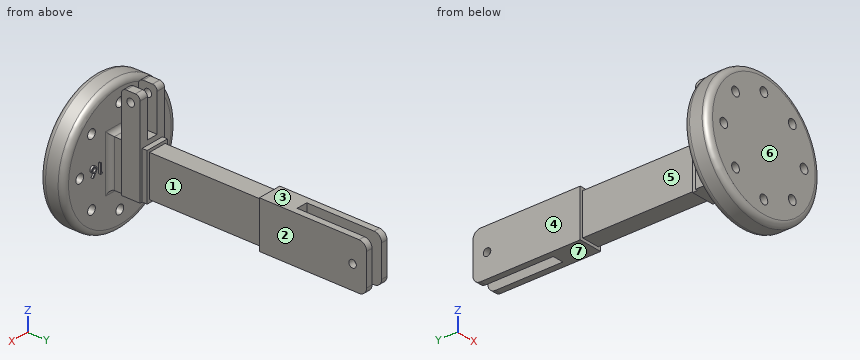
```python
from build123d import *

# Parameters (mm, degrees)
SKETCH1_W               = 70
SKETCH1_H               = 70
BOSS_EXTRUDE1_DEPTH     = 12.7
SKETCH2_R               = 2
BOSS_EXTRUDE2_DEPTH     = 6.35
CUT_EXTRUDE2_DEPTH      = 158.955689989
CUT_EXTRUDE2_DEPTH_BACK = 12.7
SKETCH3_R               = 2.413
SKETCH4_R               = 2.032
BOSS_EXTRUDE4_DEPTH     = 7.6
CUT_EXTRUDE3_DEPTH      = 12.45
SKETCH6_W               = 6
SKETCH6_H               = 36
SKETCH6_H_2             = 4
CUT_EXTRUDE4_DEPTH      = 162.187003198
BOSS_EXTRUDE5_DEPTH     = 1
SKETCH8_OUTSIDE_W       = 108.142
SKETCH8_OUTSIDE_H       = 110.642
SKETCH8_OUTSIDE_R       = 35
CUT_EXTRUDE5_DEPTH      = 147.569232812
FILLET2_R               = 3
CUT_EXTRUDE6_START      = 20
SKETCH9_OUTSIDE_W       = 108.142
SKETCH9_OUTSIDE_H       = 110.642
SKETCH9_OUTSIDE_W_2     = 9.7
SKETCH9_OUTSIDE_H_2     = 22
CUT_EXTRUDE6_DEPTH      = 60
FILLET1_R               = 2.5


with BuildPart() as part:
    # Sketch1 → Boss-Extrude1 (new body)
    with BuildSketch(Plane(origin=(0, 0, 0), x_dir=(1, 0, 0), z_dir=(0, 1, 0))):
        Rectangle(SKETCH1_W, SKETCH1_H)
    extrude(amount=BOSS_EXTRUDE1_DEPTH)

    # Sketch2 → Boss-Extrude2 (add, symmetric)
    with BuildSketch(Plane(origin=(0, 0, 0), x_dir=(0, 0, -1), z_dir=(1, 0, 0))):
        with BuildLine():
            Line((-12.5, 0), (12.5, 0))
            Line((12.5, 0), (12.5, 146))
            ThreePointArc((12.5, 146), (11.328427125, 148.828427125), (8.5, 150))
            Line((8.5, 150), (-8.5, 150))
            ThreePointArc((-8.5, 150), (-11.328427125, 148.828427125), (-12.5, 146))
            Line((-12.5, 146), (-12.5, 0))
        make_face()
        with Locations((0, 142.5)):
            Circle(SKETCH2_R, mode=Mode.SUBTRACT)
    extrude(amount=BOSS_EXTRUDE2_DEPTH, both=True)

    # Sketch3 → Cut-Extrude2 (cut, two sides: drawn at the far end of the back side and taken through both)
    with BuildSketch(Plane(origin=(0, 0, 0), x_dir=(1, 0, 0), z_dir=(0, 1, 0)).offset(-CUT_EXTRUDE2_DEPTH_BACK)):
        with Locations(Location((17.67766953, -17.67766953, 0), (0, 0, 270))):
            Circle(SKETCH3_R)
        with Locations(Location((25, 0, 0), (0, 0, 270))):
            Circle(SKETCH3_R)
        with Locations(Location((17.67766953, 17.67766953, 0), (0, 0, 270))):
            Circle(SKETCH3_R)
        with Locations(Location((0, 25, 0), (0, 0, 270))):
            Circle(SKETCH3_R)
        with Locations(Location((-17.67766953, 17.67766953, 0), (0, 0, 270))):
            Circle(SKETCH3_R)
        with Locations(Location((-25, 0, 0), (0, 0, 270))):
            Circle(SKETCH3_R)
        with Locations(Location((-17.67766953, -17.67766953, 0), (0, 0, 270))):
            Circle(SKETCH3_R)
        with Locations(Location((0, -25, 0), (0, 0, 270))):
            Circle(SKETCH3_R)
    extrude(amount=CUT_EXTRUDE2_DEPTH + CUT_EXTRUDE2_DEPTH_BACK, mode=Mode.SUBTRACT)

    # Sketch4 → Boss-Extrude4 (add, symmetric)
    with BuildSketch(Plane(origin=(0, 0, 0), x_dir=(0, 0, -1), z_dir=(1, 0, 0))):
        with BuildLine():
            Line((12.5, 20), (-35, 20))
            ThreePointArc((-35, 20), (-36.767766953, 20.732233047), (-37.5, 22.5))
            Line((-37.5, 22.5), (-37.5, 27.5))
            ThreePointArc((-37.5, 27.5), (-36.767766953, 29.267766953), (-35, 30))
            Line((-35, 30), (12.5, 30))
            Line((12.5, 30), (12.5, 20))
        make_face()
        with Locations(Location((-32.5, 25, 0), (0, 0, 180))):
            Circle(SKETCH4_R, mode=Mode.SUBTRACT)
    extrude(amount=BOSS_EXTRUDE4_DEPTH, both=True)

    # Sketch5 → Cut-Extrude3 (cut)
    with BuildSketch(Plane(origin=(0, 30, 0), x_dir=(1, 0, 0), z_dir=(0, 1, 0))):
        Polygon((-3.070505438, -14.989300838), (-3.070505438, -44.384490964), (3.070505438, -44.384490964), (2.929494562, -14.989300838), align=None)
    extrude(amount=-CUT_EXTRUDE3_DEPTH, mode=Mode.SUBTRACT)

    # Sketch6 → Cut-Extrude4 (cut, through all)
    with BuildSketch(Plane.XY.offset(12.5)):
        with Locations((0, 128)):
            Rectangle(SKETCH6_W, SKETCH6_H)
        with Locations((0, 148)):
            Rectangle(SKETCH6_W, SKETCH6_H_2)
    extrude(amount=-CUT_EXTRUDE4_DEPTH, mode=Mode.SUBTRACT)

    # Sketch7 → Boss-Extrude5 (add)
    # profile 1 of 2: a face of its own
    with BuildSketch(Plane(origin=(0, 12.7, 0), x_dir=(1, 0, 0), z_dir=(0, 1, 0))):
        Polygon((12.240261351, 2.686742079), (13.218668469, 2.686742079), (13.218668469, -2.604924587), (12.743775307, -2.604924587), (12.743775307, 2.144007037), (11.929672742, 2.144007037), align=None)
    # profile 2 of 2: a face of its own
    with BuildSketch(Plane(origin=(0, 12.7, 0), x_dir=(1, 0, 0), z_dir=(0, 1, 0))):
        with BuildLine():
            Line((17.628390691, 2.82242584), (17.994100827, 2.535157878))
            Line((17.994100827, 2.535157878), (16.595922075, 0.397078618))
            add(Edge.make_bspline(
                [(16.595922075, 0.397078618), (16.68901047, 0.411916241), (16.870589909, 0.440858701), (17.05438597, 0.445633214), (17.143957264, 0.447960028)],
                knots=[0, 0, 0, 0, 1.025318673, 2, 2, 2, 2], degree=3))
            add(Edge.make_bspline(
                [(17.143957264, 0.447960028), (17.197739491, 0.446514478), (17.303608204, 0.443668956), (17.459042297, 0.421770754), (17.60840176, 0.387261358), (17.751067531, 0.336956876), (17.887551682, 0.272697364), (18.018637448, 0.195682644), (18.141860725, 0.10193596), (18.258808341, -0.002786056), (18.364985024, -0.118774831), (18.458989298, -0.241845899), (18.537951234, -0.371871041), (18.602016567, -0.508784397), (18.65176561, -0.652374921), (18.688032645, -0.802458894), (18.709470839, -0.959139809), (18.712381997, -1.065696098), (18.713860777, -1.119823425)],
                knots=[0, 0, 0, 0, 1.04369286, 2.054478336, 3.041073146, 4.015093852, 4.984733326, 5.965804835, 6.960378782, 7.985147595, 9.009457201, 10.008161701, 10.986880575, 11.956520048, 12.937015923, 13.931873656, 14.949455224, 16, 16, 16, 16], degree=3))
            add(Edge.make_bspline(
                [(18.713860777, -1.119823425), (18.711709178, -1.193876073), (18.70747534, -1.339594158), (18.665287458, -1.551830369), (18.599731804, -1.754021196), (18.506027684, -1.942938491), (18.389637653, -2.118323329), (18.247703673, -2.273725163), (18.085259352, -2.412321529), (17.901582883, -2.528219037), (17.703911973, -2.622868888), (17.496248834, -2.690852051), (17.280610172, -2.73270682), (17.134250824, -2.737954041), (17.060214943, -2.740608348)],
                knots=[0, 0, 0, 0, 1.031375318, 2.029502543, 3.004789286, 3.987476834, 4.960371455, 5.9300674, 6.912260825, 7.929083631, 8.949397511, 9.960523116, 10.96833055, 12, 12, 12, 12], degree=3))
            add(Edge.make_bspline(
                [(17.060214943, -2.740608348), (16.989009217, -2.738297846), (16.847963141, -2.733721147), (16.640480226, -2.692951218), (16.441115902, -2.626870241), (16.251266957, -2.535831986), (16.075401269, -2.420839711), (15.918063938, -2.282406265), (15.780039469, -2.123490764), (15.665173078, -1.944117858), (15.574067614, -1.751365184), (15.505744751, -1.550376865), (15.465836145, -1.341885226), (15.460259398, -1.200550646), (15.45745052, -1.12936369)],
                knots=[0, 0, 0, 0, 1.012016664, 2.004627821, 2.994792927, 3.992885782, 4.990978636, 5.973936114, 6.964471063, 7.975201453, 8.993600317, 9.990122807, 10.98767138, 12, 12, 12, 12], degree=3))
            add(Edge.make_bspline(
                [(15.45745052, -1.12936369), (15.459236753, -1.074867713), (15.462883898, -0.96359734), (15.4883495, -0.795074346), (15.529268892, -0.622639972), (15.575095098, -0.476356846), (15.62351477, -0.356520973), (15.663810872, -0.259904982), (15.713966794, -0.160480502), (15.767447978, -0.054838219), (15.829068482, 0.05429928), (15.896069523, 0.168756019), (15.970303519, 0.286711695), (16.022343527, 0.366758276), (16.048946914, 0.407678912)],
                knots=[0, 0, 0, 0, 1.173818275, 2.396712641, 3.66331629, 4.989737886, 5.693666774, 6.447286557, 7.243889047, 8.091586357, 8.998013824, 9.943181721, 10.948533338, 12, 12, 12, 12], degree=3))
            Line((16.048946914, 0.407678912), (17.628390691, 2.82242584))
        make_face()
        with BuildLine():
            add(Edge.make_bspline(
                [(17.044314503, -0.094775015), (17.004003728, -0.095951343), (16.925265074, -0.098249053), (16.80974434, -0.111591993), (16.700413591, -0.136718438), (16.595824353, -0.168719916), (16.497931993, -0.21272097), (16.406025056, -0.266169523), (16.319748133, -0.329096781), (16.240004906, -0.400611254), (16.167706129, -0.478909827), (16.105444181, -0.562774462), (16.051737695, -0.650184031), (16.008071136, -0.741868872), (15.974068283, -0.837793937), (15.949472237, -0.93751804), (15.935783828, -1.041709908), (15.933506549, -1.112365001), (15.932343683, -1.148444219)],
                knots=[0, 0, 0, 0, 1.129588631, 2.206414736, 3.251139165, 4.268635594, 5.265702196, 6.250456724, 7.242448911, 8.251968645, 9.246821453, 10.222880186, 11.173611482, 12.116736599, 13.062300278, 14.020270554, 14.989073742, 16, 16, 16, 16], degree=3))
            add(Edge.make_bspline(
                [(15.932343683, -1.148444219), (15.933290682, -1.184200736), (15.935147605, -1.254313943), (15.952008851, -1.357636274), (15.977764273, -1.457066552), (16.016076538, -1.552092184), (16.061776714, -1.644161617), (16.122109764, -1.729939965), (16.188961333, -1.814636976), (16.268871447, -1.891746343), (16.354631769, -1.96349624), (16.446255016, -2.026210432), (16.54174686, -2.079862147), (16.64239651, -2.121909878), (16.746775972, -2.156418026), (16.855754904, -2.180701453), (16.969409103, -2.194430343), (17.046398223, -2.196710588), (17.085655648, -2.197873305)],
                knots=[0, 0, 0, 0, 0.989467248, 1.94019797, 2.891935182, 3.827694429, 4.772920941, 5.730924762, 6.725747692, 7.756678648, 8.79901574, 9.819492441, 10.826891316, 11.826466727, 12.835195252, 13.867842842, 14.912794438, 16, 16, 16, 16], degree=3))
            add(Edge.make_bspline(
                [(17.085655648, -2.197873305), (17.124913009, -2.196710497), (17.201902004, -2.194430073), (17.315557116, -2.180702479), (17.424532669, -2.156414261), (17.528924415, -2.121923525), (17.629528721, -2.07981152), (17.72493705, -2.026544213), (17.81569381, -1.963110559), (17.901510431, -1.891868959), (17.981087933, -1.814198099), (18.049542867, -1.730696019), (18.108028231, -1.643468344), (18.155553728, -1.552454868), (18.193444014, -1.457009095), (18.219330042, -1.357651667), (18.236156467, -1.254309913), (18.238018175, -1.184199375), (18.238967614, -1.148444219)],
                knots=[0, 0, 0, 0, 1.087397944, 2.132534446, 3.165364764, 4.174271784, 5.174024072, 6.181601208, 7.194203697, 8.236725232, 9.267838612, 10.269026844, 11.221737037, 12.171628256, 13.107553087, 14.05945871, 15.010357665, 16, 16, 16, 16], degree=3))
            add(Edge.make_bspline(
                [(18.238967614, -1.148444219), (18.238135624, -1.112317933), (18.236502697, -1.041413784), (18.218033346, -0.937564647), (18.19241809, -0.837287252), (18.153738984, -0.741211829), (18.103488494, -0.64971751), (18.042281438, -0.562342114), (17.971475052, -0.478415755), (17.889684724, -0.4004577), (17.800648299, -0.329175808), (17.705979497, -0.266251003), (17.60693768, -0.213145383), (17.503623267, -0.168835836), (17.39485248, -0.136859845), (17.282381372, -0.111681728), (17.164771446, -0.098283201), (17.08497824, -0.095959305), (17.044314503, -0.094775015)],
                knots=[0, 0, 0, 0, 0.978206639, 1.919901502, 2.851605144, 3.780102724, 4.718870031, 5.675451981, 6.667674623, 7.690630536, 8.733308323, 9.756129687, 10.767539656, 11.776269907, 12.797430371, 13.836405707, 14.897401972, 16, 16, 16, 16], degree=3))
        make_face(mode=Mode.SUBTRACT)
    extrude(amount=BOSS_EXTRUDE5_DEPTH)

    # Sketch8 outside → Cut-Extrude5 (cut, through all)
    with BuildSketch(Plane(origin=(0, 12.7, 0), x_dir=(1, 0, 0), z_dir=(0, 1, 0))):
        with Locations((0, -1.25)):
            Rectangle(SKETCH8_OUTSIDE_W, SKETCH8_OUTSIDE_H)
        with Locations(Location((0, 0, 0), (0, 0, 270))):
            Circle(SKETCH8_OUTSIDE_R, mode=Mode.SUBTRACT)
    extrude(amount=-CUT_EXTRUDE5_DEPTH, mode=Mode.SUBTRACT)

    # Fillet2
    fillet2_edges = [part.edges().sort_by_distance(p)[0] for p in [
        (0, 0, -35),
        (0, 12.7, -35),
    ]]
    fillet(fillet2_edges, radius=FILLET2_R)

    # Sketch9 outside → Cut-Extrude6 (cut)
    with BuildSketch(Plane(origin=(0, 12.7, 0), x_dir=(1, 0, 0), z_dir=(0, 1, 0)).offset(CUT_EXTRUDE6_START)):
        with Locations((0, -1.25)):
            Rectangle(SKETCH9_OUTSIDE_W, SKETCH9_OUTSIDE_H)
        Rectangle(SKETCH9_OUTSIDE_W_2, SKETCH9_OUTSIDE_H_2, mode=Mode.SUBTRACT)
    extrude(amount=CUT_EXTRUDE6_DEPTH, mode=Mode.SUBTRACT)

    # Fillet1
    fillet1_edges = [part.edges().sort_by_distance(p)[0] for p in [
        (-6.35, 12.7, 0),
        (0, 12.7, 12.5),
        (0, 12.7, -12.5),
        (6.35, 12.7, 0),
    ]]
    fillet(fillet1_edges, radius=FILLET1_R)


solid = part.part
```
Verification items for the finished model (mm, model axes). Face numbers are marked on the shaded views. A direction names the side the tool comes from. Coordinates: 2 decimals unless noted, no trailing zeros. Order: outer loops, then holes, each group sorted by start corner. A loop starts at its lowest first (then second) coordinate and runs counter-clockwise, first axis right, second up. Notation, with made-up numbers: (50.25, 79.5) -> (94.25, 79.5) arc R30 ccw to (94.25, 104.5) -> close; hole circle Ø11 at (54.25, 41). An arc over 180 degrees is marked (long way). Put each result on its own line as item: value. Start each with the question number.
1) Cross-section at A-A (y = 142.5). Enter the section's corners in (x, z).
2) Release check for a two-part mould opening along Y. For the marked faces 5, 6 and 7 record: pulls with the +Y half, pulls with the -Y half, needs draft (parallel to the pull), parting line crosses it, or undercut.
3) Go/stop test with flat-tipped pins: pin 1 (3.5 mm diameter, centred on x = 17, z = -0.5, fed in from +Y); pin 2 (5 mm diameter, centred on y = 27.5, z = 16.5, fed in from -X); pin 3 (1.8 mm diameter, centred on x = -0.5, z = 3.5, fed in from +Y). Record where each tip stops, or that it passes through.
4) Tool access check on the marked faces 1, 2, 3 and 4. Record the directions out of +Z, -Z, +X, -X, +Y, -Y that give a thin tool (end or side, any length) a straight path to the whole face; none if there is none.
5) Cross-section at B-B (z = 25). State how many separate pieces and enclosed holes the cut face has, plus the area to 3 significant figures.
6) Material ranges on L1, parallel to Z at x = 4, y = 25; L2, parallel to X at y = 7, z = 0; L3, parallel to X at y = 143.5, z = 3, recorded low to high.
7) Cross-section at C-C (y = 54). Enter the section's corners in (x, z), plus the area to 3 significant figures.
Geometry check:
1. outline: (-6.35, -12.5) -> (-3, -12.5) -> (-3, -2) -> (-6.35, -2) -> close; (-6.35, 2) -> (-3, 2) -> (-3, 12.5) -> (-6.35, 12.5) -> close; (3, -12.5) -> (6.35, -12.5) -> (6.35, -2) -> (3, -2) -> close; (3, 2) -> (6.35, 2) -> (6.35, 12.5) -> (3, 12.5) -> close
2. face 5: undercut
2. face 6: pulls with the -Y half
2. face 7: needs draft
3. pin 1: stops at y = 13.7
3. pin 2: stops at x = -7.6
3. pin 3: stops at y = 110
4. face 1: +Z, -Z, +X
4. face 2: +Z, -Z, +X, +Y
4. face 3: +Z, +X, -X, +Y
4. face 4: +Z, -Z, -X, +Y
5. separate pieces: 4
5. enclosed holes: 0
5. area: 641 mm^2
6. L1: z = -12.5 to 30.47, 34.53 to 37.5
6. L2: x = -35 to -27.41, -22.59 to 22.59, 27.41 to 35
6. L3: x = -6.35 to -3, 3 to 6.35
7. outline: (-4.85, -11) -> (4.85, -11) -> (4.85, 11) -> (-4.85, 11) -> close
7. area: 213 mm^2
